The model under review builds one solid part; all positions refer to its coordinate system, in mm. A direction names the side the tool comes from. Coordinates: 2 decimals unless noted, no trailing zeros. Write each loop counter-clockwise with the first axis right and the second up, starting at its lowest first coordinate (ties: lowest second). Pieces come first, ordered by that corner, then holes.
```python
from build123d import *

# Parameters (mm, degrees)
SKETCH1_R           = 8.5
BOSS_EXTRUDE1_DEPTH = 1
BOSS_EXTRUDE2_START = -7.35
BOSS_EXTRUDE2_DEPTH = 7.35


with BuildPart() as part:
    # Sketch1 → Boss-Extrude1 (new body)
    # profile 1 of 3: a face of its own
    with BuildSketch(Plane.XY.offset(55.098344014)):
        with BuildLine():
            Line((37.502628192, 13.761312554), (37.502628192, 29.761312554))
            ThreePointArc((37.502628192, 29.761312554), (25.502628192, 41.761312554), (13.502628192, 29.761312554))
            Line((13.502628192, 29.761312554), (13.502628192, 13.761312554))
            Line((13.502628192, 13.761312554), (37.502628192, 13.761312554))
        make_face()
        with BuildLine():
            ThreePointArc((35.502628192, 29.761312554), (25.502628192, 39.761312554), (15.502628192, 29.761312554))
            Line((15.502628192, 29.761312554), (15.502628192, 15.761312554))
            Line((15.502628192, 15.761312554), (35.502628192, 15.761312554))
            Line((35.502628192, 15.761312554), (35.502628192, 29.761312554))
        make_face(mode=Mode.SUBTRACT)
    # profile 2 of 3: a face of its own
    with BuildSketch(Plane.XY.offset(55.098344014)):
        with BuildLine():
            Line((35.502628192, 15.761312554), (35.502628192, 29.761312554))
            ThreePointArc((35.502628192, 29.761312554), (25.502628192, 39.761312554), (15.502628192, 29.761312554))
            Line((15.502628192, 29.761312554), (15.502628192, 15.761312554))
            Line((15.502628192, 15.761312554), (35.502628192, 15.761312554))
        make_face()
        with Locations((25.502628192, 29.761312554)):
            Circle(SKETCH1_R, mode=Mode.SUBTRACT)
    # profile 3 of 3: a face of its own
    with BuildSketch(Plane.XY.offset(55.098344014)):
        with Locations((25.502628192, 29.761312554)):
            Circle(SKETCH1_R)
    extrude(amount=BOSS_EXTRUDE1_DEPTH)

    # Sketch1<4> → Boss-Extrude2 (add)
    with BuildSketch(Plane.XY.offset(55.098344014).offset(BOSS_EXTRUDE2_START)):
        with BuildLine():
            Line((13.502628192, 29.761312554), (13.502628192, 13.761312554))
            Line((13.502628192, 13.761312554), (37.502628192, 13.761312554))
            Line((37.502628192, 13.761312554), (37.502628192, 29.761312554))
            ThreePointArc((37.502628192, 29.761312554), (25.502628192, 41.761312554), (13.502628192, 29.761312554))
        make_face()
        with BuildLine():
            Line((15.502628192, 29.761312554), (15.502628192, 15.761312554))
            Line((15.502628192, 15.761312554), (35.502628192, 15.761312554))
            Line((35.502628192, 15.761312554), (35.502628192, 29.761312554))
            ThreePointArc((35.502628192, 29.761312554), (25.502628192, 39.761312554), (15.502628192, 29.761312554))
        make_face(mode=Mode.SUBTRACT)
    extrude(amount=BOSS_EXTRUDE2_DEPTH)


solid = part.part
```
Item 1: For pin 1 (2 mm diameter, centred on x = 23.5, z = 50.5, fed in from +Y); pin 2 (1 mm diameter, centred on x = 19.5, z = 54, fed in from +Y); pin 3 (1.5 mm diameter, centred on y = 32.5, z = 50, fed in from -X); pin 4 (8 mm diameter, centred on x = 22.5, y = 37.5, fed in from -Z), all flat-tipped, find the tip position at first contact; note any pin that passes through.
Solved:
pin 1: stops at y = 41.72
pin 2: stops at y = 40.43
pin 3: stops at x = 13.67
pin 4: stops at z = 47.75
Item 2: Take a section at A-A, the plane z = 51.5. Write out the cut boundary in (x, y).
Solved:
outline: (13.5, 13.76) - (37.5, 13.76) - (37.5, 29.76) arc R12 ccw to (13.5, 29.76) - close; hole (15.5, 15.76) - (35.5, 15.76) - (35.5, 29.76) arc R10 ccw to (15.5, 29.76) - close
Item 3: Take a section at C-C, the plane x = 22.5. Write out the cut boundary in (y, z).
Solved:
outline: (13.76, 47.75) - (15.76, 47.75) - (15.76, 55.1) - (39.3, 55.1) - (39.3, 47.75) - (41.38, 47.75) - (41.38, 56.1) - (13.76, 56.1) - close
Item 4: Machinability: for faces 5 (the face through (13.503, 22, 52)), 6 (the face through (35.503, 23, 51)), which of the approach directions +Z, -Z, +X, -X, +Y, -Y give a long, thin tool a straight path to every point of the face, cutting with its end or side? Answer none if there is none.
Solved:
face 5: +Z, -Z, -X, +Y, -Y
face 6: -Z
Item 5: Mouldability with a two-part tool opening along Y and no side actions: class faces 1 (the face through (25, 13.761, 52)), 2 (the face through (25, 28, 56.098)), 3 (the face through (15.503, 23, 51)), 4 (the face through (25.77, 41.76, 51.86)) as pulls with the +Y half, pulls with the -Y half, needs draft (parallel to the pull), parting line crosses it, or undercut.
Solved:
face 1: pulls with the -Y half
face 2: needs draft
face 3: undercut
face 4: pulls with the +Y half
Item 6: To check wall thickness, follow line 1 along X through (y, z) = (19.75, 53); line 2 along Z through (x, y) = (31.5, 23.75); line 3 along Y through (x, z) = (31, 50.75). State the ranges of each line that lie inside material, in increasing order.
Solved:
line 1: x = 13.5 to 15.5, 35.5 to 37.5
line 2: z = 55.1 to 56.1
line 3: y = 13.76 to 15.76, 38.11 to 40.43
Item 7: Take a section at B-B, the plane y = 22. Write out the cut boundary in (x, z).
Solved:
outline: (13.5, 47.75) - (15.5, 47.75) - (15.5, 55.1) - (35.5, 55.1) - (35.5, 47.75) - (37.5, 47.75) - (37.5, 56.1) - (13.5, 56.1) - close
